Input: part model. Units: mm. Frame: model coordinates. A direction names the side the tool comes from. Give positions to 0.01 mm unless a question says otherwise; leave off trailing zeros. Order: outer loops, then holes, each group sorted by start corner. A loop starts at its lowest first (then second) coordinate and runs counter-clockwise, first axis right, second up.
```python
from build123d import *

# Parameters (mm, degrees)
SKETCH1_W               = 265
SKETCH1_H               = 170
BOSS_EXTRUDE1_DEPTH     = 18
CUT_EXTRUDE1_DEPTH      = 1
CUT_EXTRUDE1_DEPTH_BACK = 266
BOSS_EXTRUDE2_DEPTH     = 265
SKETCH4_W               = 253
SKETCH4_H               = 92.678428724
BOSS_EXTRUDE3_DEPTH     = 2
BOSS_EXTRUDE4_DEPTH     = 265
SKETCH8_R               = 8.5
CUT_EXTRUDE3_DEPTH      = 17


with BuildPart() as part:
    # Sketch1 → Boss-Extrude1 (new body)
    with BuildSketch(Plane(origin=(0, 0, 0), x_dir=(1, 0, 0), z_dir=(0, 1, 0))):
        Rectangle(SKETCH1_W, SKETCH1_H)
    extrude(amount=BOSS_EXTRUDE1_DEPTH)

    # Sketch2 → Cut-Extrude1 (cut, two sides)
    with BuildSketch(Plane(origin=(132.5, 0, 0), x_dir=(0, 0, -1), z_dir=(1, 0, 0))) as cut_extrude1_sk:
        with BuildLine():
            Line((-266.258489167, 313.568151134), (-85, 13))
            ThreePointArc((-85, 13), (-76.493710292, 4.201984165), (-65, 0))
            Line((-65, 0), (283.270913158, -43.625960377))
            Line((283.270913158, -43.625960377), (-99.302917842, -632.201084994))
            Line((-99.302917842, -632.201084994), (-648.832320167, -275.006973483))
            Line((-648.832320167, -275.006973483), (-266.258489167, 313.568151134))
        make_face()
    extrude(amount=CUT_EXTRUDE1_DEPTH, mode=Mode.SUBTRACT)
    extrude(cut_extrude1_sk.sketch, amount=-CUT_EXTRUDE1_DEPTH_BACK, mode=Mode.SUBTRACT)

    # Sketch3 → Boss-Extrude2 (add)
    with BuildSketch(Plane.ZY.offset(132.5)):
        with BuildLine():
            ThreePointArc((-85, 15), (-88.140347905, 8.402718027), (-95.24097163, 6.680203261))
            add(Edge.make_bspline(
                [(-95.24097163, 6.680203261), (-89.327681397, 4.618052191), (-85, 0)],
                knots=[0, 0, 0, 1, 1, 1], degree=2))
            Line((-85, 0), (-85, 15))
        make_face()
        with BuildLine():
            add(Edge.make_bspline(
                [(-86.53925872, 19.878327668), (-86.439507091, 19.716554468), (-86.33208607, 19.568480042)],
                knots=[0, 0, 0, 0.074961469, 0.074961469, 0.074961469], degree=2))
            ThreePointArc((-86.53925872, 19.878327668), (-100.596416051, 19.678768987), (-95.24097163, 6.680203261))
            ThreePointArc((-95.24097163, 6.680203261), (-88.140347905, 8.402718027), (-85, 15))
            ThreePointArc((-85, 15), (-85.339814083, 17.379362477), (-86.33208607, 19.568480042))
        make_face()
        with BuildLine():
            add(Edge.make_bspline(
                [(-86.33208607, 19.568480042), (-85.335385171, 18.194578424), (-83.678428785, 18)],
                knots=[0.074961469, 0.074961469, 0.074961469, 0.770487944, 0.770487944, 0.770487944], degree=2))
            ThreePointArc((-86.33208607, 19.568480042), (-85.339814083, 17.379362477), (-85, 15))
            Line((-85, 15), (-85, 18))
            Line((-85, 18), (-83.678428785, 18))
        make_face()
    extrude(amount=-BOSS_EXTRUDE2_DEPTH)

    # Sketch4 → Boss-Extrude3 (add)
    with BuildSketch(Plane(origin=(0, 18, 0), x_dir=(1, 0, 0), z_dir=(0, 1, 0))):
        with Locations((0, 24.339214362)):
            Rectangle(SKETCH4_W, SKETCH4_H)
    extrude(amount=BOSS_EXTRUDE3_DEPTH)

    # Sketch6 → Boss-Extrude4 (add)
    with BuildSketch(Plane.ZY.offset(132.5)):
        with BuildLine():
            Line((-101.203779097, 11.408094152), (-78.679249537, 0))
            add(Edge.make_bspline(
                [(-89, -7.5), (-87.236541116, 0.615126939), (-78.679249537, 0)],
                knots=[0, 0, 0, 1, 1, 1], degree=2))
            ThreePointArc((-89, -7.5), (-106.371084282, -17.388395692), (-106.005281627, 2.596626873))
            add(Edge.make_bspline(
                [(-106.005281627, 2.596626873), (-101.037094557, 5.737965522), (-101.203779097, 11.408094152)],
                knots=[0, 0, 0, 1, 1, 1], degree=2))
        make_face()
    extrude(amount=-BOSS_EXTRUDE4_DEPTH)

    # Sketch8 → Cut-Extrude3 (cut)
    with BuildSketch(Plane.ZY.offset(132.5)):
        with Locations((-93.5, 15)):
            Circle(SKETCH8_R)
    cut_extrude3 = extrude(amount=-CUT_EXTRUDE3_DEPTH, mode=Mode.SUBTRACT)

    # Mirror1: Cut-Extrude3 across plane
    add(cut_extrude3.mirror(Plane(origin=(0, 0, 0), x_dir=(0, 0, 1), z_dir=(1, 0, 0))), mode=Mode.SUBTRACT)


solid = part.part
```
1) Cut plane C-C (z = 29). Return the cut outline in (x, y).
2) First-contact query: P1, Ø4, axis at x = 64.5, y = -4.5, coming from the +Z side; P2, Ø3, axis at x = 48.5, z = -2.5, coming from the -Y side; P3, Ø2, axis at y = 19.5, z = -30, coming from the -X side. Flat tips, straight axial feed; report the tip coordinate or a pass-through.
3) Pull-direction query (Y, two-part tool) for faces 4 (the face through (-2, 20, -25)), 5 (the face through (-132.5, 9, -15)), 6 (the face through (124.12, 7.46, -89.58)); classes: pulls with the +Y half, pulls with the -Y half, needs draft (parallel to the pull), parting line crosses it, or undercut.
4) Cut plane B-B (z = -93.5). Return the cut outline in (x, y).
5) Line query: probe 1 along Y at (x, z) = (8, -29); probe 2 along Z at (x, y) = (87.5, 16); probe 3 along Z at (x, y) = (68.5, -8.5). Output: solid intervals per line, ascending.
6) Reachability of faces 1 (the face through (-2, 15, 85)), 2 (the face through (-124.12, 7.46, -89.58)), 3 (the face through (-2, 0, -9)) from +Z, -Z, +X, -X, +Y, -Y: full face, straight path, thin tool, end or side. Return the list, or none.
7) Cut plane A-A (z = -59). Return the cut outline in (x, y).
Geometry says:
1. outline: (-132.5, 0) - (132.5, 0) - (132.5, 18) - (-132.5, 18) - close
2. P1: stops at z = -86.59
2. P2: stops at y = 0
2. P3: stops at x = -126.5
3. face 4: pulls with the +Y half
3. face 5: needs draft
3. face 6: undercut
4. outline: (-132.5, -16.62) - (132.5, -16.62) - (132.5, 6.5) - (115.5, 6.5) - (115.5, 23.5) - (-115.5, 23.5) - (-115.5, 6.5) - (-132.5, 6.5) - close
5. probe 1: y = 0 to 20
5. probe 2: z = -101.94 to 85
5. probe 3: z = -111.96 to -89.04
6. face 1: +Z, +X, -X, +Y, -Y
6. face 2: -X
6. face 3: +Z, +X, -X, -Y
7. outline: (-132.5, 0) - (132.5, 0) - (132.5, 18) - (126.5, 18) - (126.5, 20) - (-126.5, 20) - (-126.5, 18) - (-132.5, 18) - close
